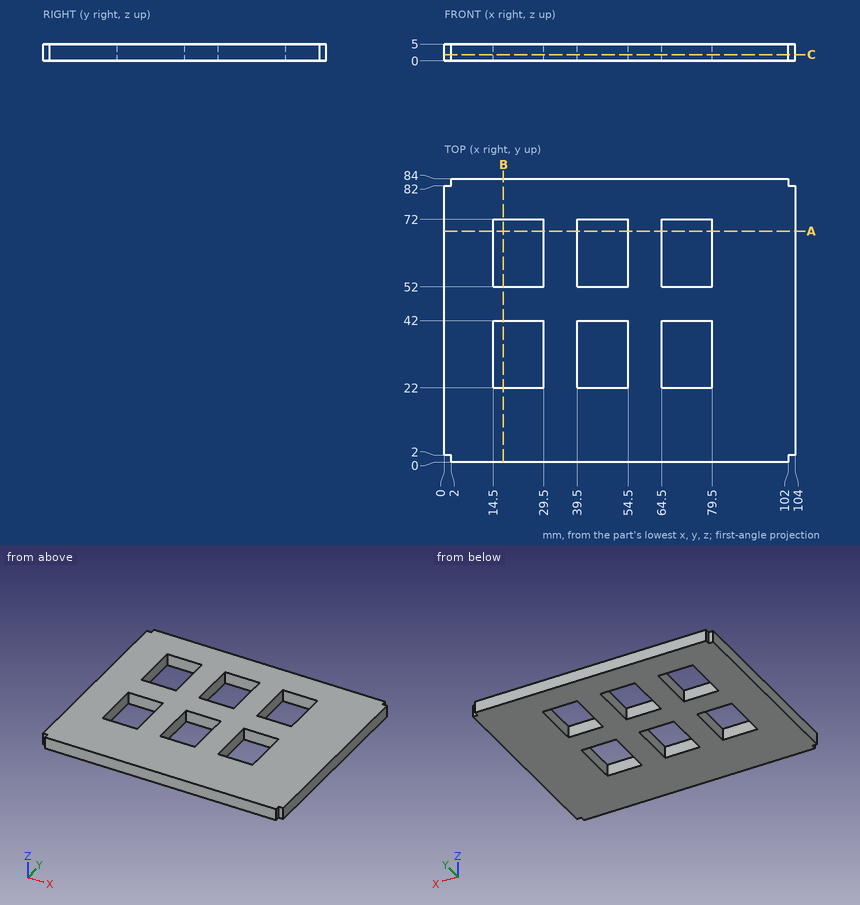
Drawing for the job (mm, zero at the part's lowest x, y, z). Give positions to 0.01 mm unless a question says otherwise; leave off trailing zeros. Loops run counter-clockwise (first coordinate to the right, second up) from the corner with the lowest first, then second, coordinate; pieces in that order, holes last. Notation, with made-up numbers: (36, -15.5) - (50, -15.5) arc R23 ccw to (50, -3.5) - close; hole circle Ø4 at (-0.75, 16.5). An arc over 180 degrees is marked (long way). Write item = value, one per line. Start each with the question number.
1) Band-saw the part on A-A on y = 68.5. Give the cut face in (x, z).
2) Band-saw the part on B-B on x = 17.5. Give the cut face in (y, z).
3) Drop flat-ended pins along their axis: pin 1 Ø5 at (x, y) = (26, 68.5) entering from -Z; pin 2 Ø0.6 at (x, z) = (0.5, 2) entering from +Y; pin 3 Ø2 at (x, z) = (0.5, 2.5) entering from -Y. Give the stop position or say it passes through.
4) Probe probe 1 along X at (y, z) = (66, 0.3); probe 2 along Y at (x, z) = (19.5, 1.15). List the from-to ranges inside material, lowest first. Write a range as from..to.
5) Band-saw the part on C-C on z = 1.85. Count the separate pieces of the cut face and the enclosed holes in it, plus the area to 3 significant figures.
Final values:
q1.outline = (0, 0) - (14.5, 0) - (14.5, 5) - (0, 5) - close; (29.5, 0) - (39.5, 0) - (39.5, 5) - (29.5, 5) - close; (54.5, 0) - (64.5, 0) - (64.5, 5) - (54.5, 5) - close; (79.5, 0) - (104, 0) - (104, 5) - (79.5, 5) - close
q2.outline = (0, 0) - (22, 0) - (22, 5) - (0, 5) - close; (42, 0) - (52, 0) - (52, 5) - (42, 5) - close; (72, 0) - (84, 0) - (84, 5) - (72, 5) - close
q3.pin_1 = through
q3.pin_2 = 82
q3.pin_3 = 2
q4.probe_1 = 0..14.5, 29.5..39.5, 54.5..64.5, 79.5..104
q4.probe_2 = 0..22, 42..52, 72..84
q5.separate_pieces = 1
q5.enclosed_holes = 6
q5.area = 6,920 mm²
